```python
from build123d import *

# Parameters (mm, degrees)
SKETCH3_R           = 18.415
BOSS_EXTRUDE1_DEPTH = 1.016
SKETCH5_R           = 19.304
BOSS_EXTRUDE2_DEPTH = 0.508
SKETCH6_R           = 19.558
BOSS_EXTRUDE3_DEPTH = 2.54
SKETCH7_R           = 15.24
BOSS_EXTRUDE4_DEPTH = 1.27
SKETCH8_R           = 1.524
SKETCH8_R_2         = 1.27
BOSS_EXTRUDE5_DEPTH = 0.635
CIRPATTERN1_COUNT   = 12
SKETCH9_W           = 20.32
SKETCH9_H           = 12.7
BOSS_EXTRUDE6_DEPTH = 19.05
BOSS_EXTRUDE7_DEPTH = 20.32
SKETCH12_R          = 3.81
BOSS_EXTRUDE8_DEPTH = 3.048
SKETCH13_R          = 5.08
BOSS_EXTRUDE9_DEPTH = 1.524


with BuildPart() as part:
    # Sketch1 → Revolve3 (revolve)
    with BuildSketch(Plane(origin=(0, 0, 0), x_dir=(1, 0, 0), z_dir=(0, 1, 0))):
        with BuildLine():
            Line((0, 0), (0, -12.7))
            Line((0, -12.7), (-19.05, -12.7))
            ThreePointArc((-19.05, -12.7), (-17.408709569, -5.583145216), (-12.7, 0))
            Line((-12.7, 0), (0, 0))
        make_face()
    revolve(axis=Axis((0, 0, 0), (0, 0, 1)))

    # Sketch3 → Boss-Extrude1 (add)
    with BuildSketch(Plane.XY.offset(12.7)):
        Circle(SKETCH3_R)
    extrude(amount=BOSS_EXTRUDE1_DEPTH)

    # Sketch4 → Revolve4 (revolve)
    with BuildSketch(Plane(origin=(0, 0, 0), x_dir=(1, 0, 0), z_dir=(0, 1, 0))):
        with BuildLine():
            Line((0, -13.716), (-18.796, -13.716))
            ThreePointArc((-18.796, -13.716), (-19.781066859, -18.796), (-18.796, -23.876))
            Line((-18.796, -23.876), (0, -23.876))
            Line((0, -23.876), (0, -13.716))
        make_face()
    revolve(axis=Axis((0, 0, 23.876), (0, 0, -1)))

    # Sketch5 → Boss-Extrude2 (add)
    with BuildSketch(Plane.XY.offset(23.876)):
        Circle(SKETCH5_R)
    extrude(amount=BOSS_EXTRUDE2_DEPTH)

    # Sketch6 → Boss-Extrude3 (add)
    with BuildSketch(Plane.XY.offset(24.384)):
        Circle(SKETCH6_R)
    extrude(amount=BOSS_EXTRUDE3_DEPTH)

    # Sketch7 → Boss-Extrude4 (add)
    with BuildSketch(Plane.XY.offset(26.924)):
        Circle(SKETCH7_R)
    extrude(amount=BOSS_EXTRUDE4_DEPTH)

    # Sketch8 → Boss-Extrude5 (add)
    with BuildSketch(Plane.XY.offset(26.924)):
        with Locations((17.399, 0)):
            Circle(SKETCH8_R)
        with Locations((17.399, 0)):
            Circle(SKETCH8_R_2, mode=Mode.SUBTRACT)
    boss_extrude5 = extrude(amount=BOSS_EXTRUDE5_DEPTH)

    # CirPattern1: Boss-Extrude5 ×12 about axis
    cirpattern1_axis = Axis((0, 0, 0), (0, 0, 1))
    for i in range(1, CIRPATTERN1_COUNT):
        add(boss_extrude5.rotate(cirpattern1_axis, i * 360 / CIRPATTERN1_COUNT))

    # Sketch9 → Boss-Extrude6 (add)
    with BuildSketch(Plane(origin=(0, 0, 0), x_dir=(-1, 0, 0), z_dir=(0, 0, -1))):
        Rectangle(SKETCH9_W, SKETCH9_H)
    extrude(amount=BOSS_EXTRUDE6_DEPTH)

    # Sketch10 → Boss-Extrude7 (add)
    with BuildSketch(Plane(origin=(10.16, 0, 0), x_dir=(0, 0, -1), z_dir=(1, 0, 0))):
        with BuildLine():
            Line((19.05, 6.35), (19.05, -6.35))
            ThreePointArc((19.05, -6.35), (21.680256121, 0), (19.05, 6.35))
        make_face()
    extrude(amount=-BOSS_EXTRUDE7_DEPTH)

    # Sketch12 → Boss-Extrude8 (add)
    with BuildSketch(Plane.XY.offset(28.194)):
        Circle(SKETCH12_R)
    extrude(amount=BOSS_EXTRUDE8_DEPTH)

    # Sketch13 → Boss-Extrude9 (add)
    with BuildSketch(Plane.ZY.offset(10.16)):
        with Locations((-12.7, 0)):
            Circle(SKETCH13_R)
    extrude(amount=BOSS_EXTRUDE9_DEPTH)


solid = part.part
```
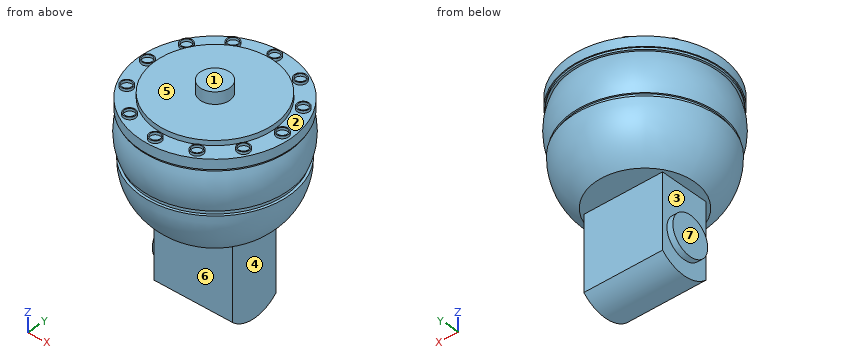
Work out the finished part from the listing and answer in its coordinate system (mm). Face numbers are marked on the shaded views. A direction names the side the tool comes from. Give positions to 0.01 mm unless a question says otherwise; leave off trailing zeros. Loops run counter-clockwise (first coordinate to the right, second up) from the corner with the lowest first, then second, coordinate; pieces in that order, holes last. Notation, with made-up numbers: M 73.25,68 L 83.25,68 A26 ccw 83.25,106 Z; hole C -11.5,39 d6. An arc over 180 degrees is marked long. One line per item, written item: value. Start each with the question number.
1. Find section A-A (z = -12.7). Give the vertices of the cut face in (x, y), and give its area (3 significant figures).
2. Determine the mould class of the marked faces 1, 2, 3 and 4 for opening direction X: released by +X, released by -X, zero draft, split by the parting line, or undercut.
3. Which of the six approach directions +Z, -Z, +X, -X, +Y, -Y give full straight-line access (tool end or side, diameter ignored) to the marked faces 5, 6 and 7?
4. Find the intervals of material crossed by probe 1 along Z at (x, y) = (4.5, 0); probe 2 along X at (y, z) = (-3, 12); probe 3 along Z at (x, y) = (-4.5, 9), in increasing order.
5. Each of these flat-tipped pins is pushed along its axis until it touches: P1, Ø2.5, axis at x = -0.5, y = 18, coming from the +Z side; P2, Ø3, axis at x = -5, z = -5, coming from the +Y side; P3, Ø3, axis at x = 8.7, y = -15.07, coming from the -Z side; P4, Ø2, axis at x = -14.5, y = 15, coming from the -Z side. Where does it stop, or does it pass through?
Reported:
1. outline: M -11.68,-5.08 L -10.16,-5.08 L -10.16,-6.35 L 10.16,-6.35 L 10.16,6.35 L -10.16,6.35 L -10.16,5.08 L -11.68,5.08 Z
1. area: 274 mm²
2. face 1: zero draft
2. face 2: undercut
2. face 3: released by -X
2. face 4: released by +X
3. face 5: +Z
3. face 6: -Z, +X, -X, -Y
3. face 7: -Z, -X, +Y, -Y
4. probe 1: z = -21.68 to 28.19
4. probe 2: x = -18.8 to 18.8
4. probe 3: z = 0 to 28.19
5. P1: stops at z = 27.56
5. P2: stops at y = 6.35
5. P3: stops at z = 3.15
5. P4: passes through
